CAD build for the part. Positions are in the model's coordinates, mm. Face numbers are marked on the shaded views. A direction names the side the tool comes from. Give positions to 0.01 mm unless a question says otherwise; leave off trailing zeros. Loops run counter-clockwise (first coordinate to the right, second up) from the corner with the lowest first, then second, coordinate; pieces in that order, holes last.
```python
from build123d import *

# Parameters (mm, degrees)
F0_W     = 114.3
F0_H     = 63.5
F1_DEPTH = 12.7
F2_W     = 114.3
F2_H     = 50.8
F3_DEPTH = 12.7
F5_DEPTH = 12.7
F7_DEPTH = 12.7


with BuildPart() as f1:
    # F0 (on Top) → F1 (new body)
    with BuildSketch(Plane.XY):
        with Locations((57.15, 31.75)):
            Rectangle(F0_W, F0_H)
    extrude(amount=F1_DEPTH)

    # F2 (on face) → F3 (join)
    with BuildSketch(Plane.XY.offset(12.7)):
        with Locations((57.15, 38.1)):
            Rectangle(F2_W, F2_H)
    extrude(amount=F3_DEPTH)

    # F4 (on face) → F5 (join)
    with BuildSketch(Plane.XY.offset(25.4)):
        Polygon((0, 12.7), (12.7, 12.7), (12.7, 44.45), (31.75, 44.45), (31.75, 57.15), (82.55, 57.15), (82.55, 44.45), (101.6, 44.45), (101.6, 12.7), (114.3, 12.7), (114.3, 63.5), (0, 63.5), align=None)
    extrude(amount=F5_DEPTH)

    # F6 (on face) → F7 (join)
    with BuildSketch(Plane.XY.offset(38.1)):
        Polygon((25.4, 63.5), (25.4, 44.45), (31.75, 44.45), (31.75, 57.15), (82.55, 57.15), (82.55, 44.45), (88.9, 44.45), (88.9, 63.5), align=None)
    extrude(amount=F7_DEPTH)


solid = f1.part
```
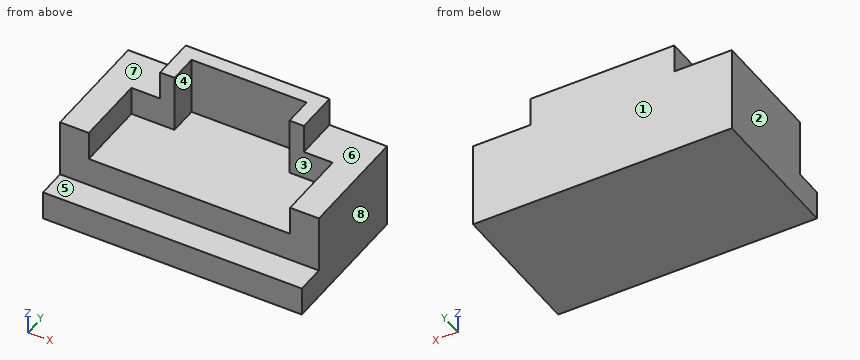
1. Pull direction X, two halves, no side cores. Call the marked faces 1, 2 and 3: released by +X, released by -X, zero draft, split by the parting line, or undercut.
Responses:
face 1: zero draft
face 2: released by -X
face 3: undercut
2. Drop flat-ended pins along their axis: pin 1 (21 mm diameter, centred on x = 90.5, z = 40.5, fed in from -Y); pin 2 (12.5 mm diameter, centred on x = 104.5, y = 48.5, fed in from +Z); pin 3 (4 mm diameter, centred on y = 48.5, z = 44.5, fed in from +X); pin 4 (8 mm diameter, centred on y = 7.5, z = 28, fed in from -X). Give the stop position or say it passes through.
Responses:
pin 1: stops at y = 44.45
pin 2: stops at z = 38.1
pin 3: stops at x = 88.9
pin 4: passes through
3. Tool access for the marked faces 4, 5, 6, 7 and 8: list every direction of +Z, -Z, +X, -X, +Y, -Y with a clear straight run to the whole face (end or side of a thin tool).
Responses:
face 4: +Z, -Y
face 5: +Z, +X, -X, -Y
face 6: +Z, +X, +Y, -Y
face 7: +Z, -X, +Y, -Y
face 8: +Z, -Z, +X, +Y, -Y
4. Saw through at C-C, the plane y = 59.5. List the corners of the cut face in (x, z).
Responses:
outline: (0, 0) - (114.3, 0) - (114.3, 38.1) - (88.9, 38.1) - (88.9, 50.8) - (25.4, 50.8) - (25.4, 38.1) - (0, 38.1) - close
5. Saw through at D-D, the plane z = 17. List the corners of the cut face in (x, y).
Responses:
outline: (0, 12.7) - (114.3, 12.7) - (114.3, 63.5) - (0, 63.5) - close
6. Probe line 1 along X through (y, z) = (24, 25.5); line 2 along X through (y, z) = (54, 30); line 3 along Z through (x, y) = (88, 24). List the from-to ranges inside material, lowest first.
Responses:
line 1: x = 0 to 12.7, 101.6 to 114.3
line 2: x = 0 to 31.75, 82.55 to 114.3
line 3: z = 0 to 25.4
7. Saw through at B-B, the plane z = 34. List the corners of the cut face in (x, y).
Responses:
outline: (0, 12.7) - (12.7, 12.7) - (12.7, 44.45) - (31.75, 44.45) - (31.75, 57.15) - (82.55, 57.15) - (82.55, 44.45) - (101.6, 44.45) - (101.6, 12.7) - (114.3, 12.7) - (114.3, 63.5) - (0, 63.5) - close
8. Saw through at A-A, the plane x = 74. List the corners of the cut face in (y, z), and give its area (3 significant figures).
Responses:
outline: (0, 0) - (63.5, 0) - (63.5, 50.8) - (57.15, 50.8) - (57.15, 25.4) - (12.7, 25.4) - (12.7, 12.7) - (0, 12.7) - close
area: 1,610 mm2
